Part model, mm, in its own coordinate system. Face numbers are marked on the shaded views. A direction names the side the tool comes from. Give positions to 0.01 mm unless a question says otherwise; leave off trailing zeros. Order: outer loops, then holes, each group sorted by start corner. A loop starts at its lowest first (then second) coordinate and runs counter-clockwise, first axis right, second up. Notation, with made-up numbers: (34.5, 3) -> (47.5, 3) arc R27 ccw to (47.5, 23) -> close; hole circle Ø10 at (14, 30). An arc over 180 degrees is marked (long way). Write item = value, one per line. Start each with the question number.
Item 1: Band-saw the part on D-D on y = 9. Count the separate pieces of the cut face and the enclosed holes in it, plus the area to 3 significant figures.
Item 2: Pull direction X, two halves, no side cores. Call the marked faces 4, 5 and 6: +X half, -X half, draft (parallel to the pull), parting line (faces both ways), or undercut.
Item 3: Band-saw the part on B-B on z = 30. Write the cut outline in (x, y).
Item 4: Tool access for the marked faces 1, 2 and 3: list every direction of +Z, -Z, +X, -X, +Y, -Y with a clear straight run to the whole face (end or side of a thin tool).
Item 5: Band-saw the part on C-C on z = 0. Write the cut outline in (x, y).
Item 6: Flat gauge pins, fed straight in: P1, Ø5, axis at x = 96, y = 6.5, coming from the -Z side; P2, Ø18.5, axis at x = 69, z = -2.5, coming from the +Y side; P3, Ø5, axis at x = 71.5, y = 10, coming from the +Z side; P4, Ø14.5, axis at y = 5.5, z = -25, coming from the +X side. Where does each tip first touch, or does it go through?
Item 7: Band-saw the part on A-A on x = 0. Write the cut outline in (y, z), plus the area to 3 significant figures.
Item 8: Drill centre lines: line 1 along X through (y, z) = (5, 31.5); line 2 along Y through (x, z) = (61.5, 17.5); line 3 along Y through (x, z) = (36, 2.5). Where is each one in solid material? Low to high.
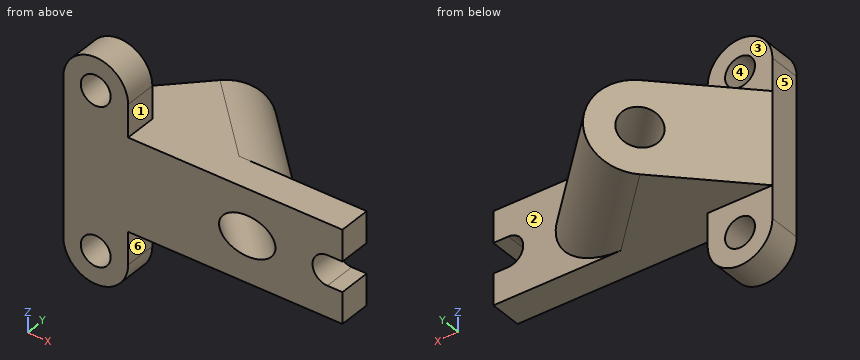
```python
from build123d import *

# Parameters (mm, degrees)
SKETCH1_R           = 6
BOSS_EXTRUDE1_DEPTH = 13
SKETCH2_W           = 86
SKETCH2_H           = 13
BOSS_EXTRUDE2_DEPTH = 18.5
CUT_EXTRUDE1_DEPTH  = 37
SKETCH4_R           = 8
BOSS_EXTRUDE3_DEPTH = 64
SKETCH6_W           = 112
SKETCH6_H           = 33.393710728
CUT_EXTRUDE2_DEPTH  = 32
SKETCH7_R           = 8
CUT_EXTRUDE3_DEPTH  = 88


with BuildPart() as part:
    # Sketch1 → Boss-Extrude1 (new body)
    with BuildSketch(Plane(origin=(0, 0, 0), x_dir=(1, 0, 0), z_dir=(0, 1, 0))):
        with BuildLine():
            Line((13, 31.5), (13, -31.5))
            ThreePointArc((13, -31.5), (0, -44.5), (-13, -31.5))
            Line((-13, -31.5), (-13, 31.5))
            ThreePointArc((-13, 31.5), (0, 44.5), (13, 31.5))
        make_face()
        with Locations(Location((0, 31.5, 0), (0, 0, 90))):
            Circle(SKETCH1_R, mode=Mode.SUBTRACT)
        with Locations(Location((0, -31.5, 0), (0, 0, 90))):
            Circle(SKETCH1_R, mode=Mode.SUBTRACT)
    extrude(amount=BOSS_EXTRUDE1_DEPTH)

    # Sketch2 → Boss-Extrude2 (add, symmetric)
    with BuildSketch(Plane.XY):
        with Locations((56, 6.5)):
            Rectangle(SKETCH2_W, SKETCH2_H)
    extrude(amount=BOSS_EXTRUDE2_DEPTH, both=True)

    # Sketch3 → Cut-Extrude1 (cut)
    with BuildSketch(Plane(origin=(0, 13, 0), x_dir=(1, 0, 0), z_dir=(0, 1, 0))):
        with BuildLine():
            Line((105, -6), (93, -6))
            ThreePointArc((93, -6), (87, 0), (93, 6))
            Line((93, 6), (105, 6))
            ThreePointArc((105, 6), (111, 0), (105, -6))
        make_face()
    extrude(amount=-CUT_EXTRUDE1_DEPTH, mode=Mode.SUBTRACT)

    # Sketch4 → Boss-Extrude3 (add)
    with BuildSketch(Plane(origin=(-13, 13, 0), x_dir=(0, 0, 1), z_dir=(-0.7071067811865488, 0.7071067811865464, 0))):
        with BuildLine():
            Line((-18.5, 43), (-18.5, 0))
            Line((-18.5, 0), (18.5, 0))
            Line((18.5, 0), (18.5, 43))
            ThreePointArc((18.5, 43), (0, 61.5), (-18.5, 43))
        make_face()
        with Locations(Location((0, 43, 0), (0, 0, 270))):
            Circle(SKETCH4_R, mode=Mode.SUBTRACT)
    extrude(amount=-BOSS_EXTRUDE3_DEPTH)

    # Sketch6 → Cut-Extrude2 (cut, symmetric)
    with BuildSketch(Plane.XY):
        with Locations((43, -16.696855364)):
            Rectangle(SKETCH6_W, SKETCH6_H)
    extrude(amount=CUT_EXTRUDE2_DEPTH, both=True, mode=Mode.SUBTRACT)

    # Sketch7 → Cut-Extrude3 (cut)
    with BuildSketch(Plane(origin=(-13, 13, 0), x_dir=(0, 0, 1), z_dir=(-0.7071067811865487, 0.7071067811865465, 0))):
        with Locations(Location((0, 43, 0), (0, 0, 270))):
            Circle(SKETCH7_R)
    extrude(amount=-CUT_EXTRUDE3_DEPTH, mode=Mode.SUBTRACT)


solid = part.part
```
Values found:
q1.separate_pieces = 1
q1.enclosed_holes = 3
q1.area = 4,710 mm^2
q2.face_4 = undercut
q2.face_5 = -X half
q2.face_6 = +X half
q3.outline = (-13, 0) -> (-5.81, 0) -> (-5.81, 13) -> (-13, 13) -> close; (5.81, 0) -> (13, 0) -> (13, 13) -> (5.81, 13) -> close
q4.face_1 = +Z, +X, +Y, -Y
q4.face_2 = +X, +Y
q4.face_3 = +Z, +X, -X, +Y
q5.outline = (-13, 0) -> (49.5, 0) -> (11.75, 37.75) -> (-13, 13) -> close; (23.06, 49.06) -> (72.12, 0) -> (87, 0) -> (87, 13) -> (73.97, 13) -> (30.49, 56.49) -> close
q6.P1 = -18.5
q6.P2 = 27.08
q6.P3 = 18.5
q6.P4 = 99
q7.outline = (0, -44.5) -> (13, -44.5) -> (13, -37.5) -> (0, -37.5) -> close; (0, -25.5) -> (13, -25.5) -> (13, -18.5) -> (26, -18.5) -> (26, 18.5) -> (13, 18.5) -> (13, 25.5) -> (0, 25.5) -> close; (0, 37.5) -> (13, 37.5) -> (13, 44.5) -> (0, 44.5) -> close
q7.area = 1,330 mm^2
q8.line_1 = -13 to -6, 6 to 13
q8.line_2 = 0 to 13
q8.line_3 = 0 to 14.06, 35.56 to 50.73
